Autodesk Inventor part; units mm, degrees
ref_plane "YZ Plane" through (0, 0, 0) normal (1, 0, 0) x (0, 1, 0)
ref_plane "XZ Plane" through (0, 0, 0) normal (0, 1, 0) x (-1, 0, 0)
ref_plane "XY Plane" through (0, 0, 0) normal (0, 0, 1) x (1, 0, 0)
sketch "スケッチ1" plane through (0, 0, 0) normal (0, 1, 0) x (-1, 0, 0)
  line L0 (-8, 10) -> (8, 10)
  line L1 (8, 10) -> (8, -10)
  line L2 (8, -10) -> (-8, -10)
  line L3 (-8, -10) -> (-8, 10)
  line L4 (-8, 10) -> (8, -10) construction
  line L5 (8, 10) -> (-8, -10) construction
  circle A0 centre (0, 15) radius 5
  circle A1 centre (0, -15) radius 5
  line L6 (4.4944, 17.191) -> (8, 10)
  line L7 (-8, 10) -> (-4.4944, 17.191)
  line L8 (4.4944, -17.191) -> (8, -10)
  line L9 (-8, -10) -> (-4.4944, -17.191)
  point P0 (0, 0)
  dimension "d0" = 16
  dimension "d1" = 20
  dimension "d2" = 10
  dimension "d3" = 10
extrude "押し出し1" add sketch "スケッチ1" along normal blind 6.5
sketch "スケッチ2" plane through (0, 6.5, 0) normal (0, 1, 0) x (1, 0, 0)
  line L0 (5.25, -7.8) -> (-5.25, -7.8)
  line L1 (-5.25, -7.8) -> (-5.25, 7.8)
  line L2 (-5.25, 7.8) -> (5.25, 7.8)
  line L3 (5.25, 7.8) -> (5.25, -7.8)
  line L4 (5.25, -7.8) -> (-5.25, 7.8) construction
  line L5 (-5.25, -7.8) -> (5.25, 7.8) construction
  point P0 (0, 0)
  dimension "d6" = 10.5
  dimension "d7" = 15.6
extrude "押し出し2" cut sketch "スケッチ2" against normal blind 1.8
sketch "スケッチ3" plane through (0, 4.7, 0) normal (0, 1, 0) x (1, 0, 0)
  line L0 (-5.25, 7.8) -> (5.25, 7.8)
  line L1 (-5.25, -7.8) -> (-5.25, 7.8)
  line L2 (5.25, -7.8) -> (-5.25, -7.8)
  line L3 (5.25, 7.8) -> (5.25, -7.8)
  line L4 (-5.25, -7.8) -> (-3.65, -7.8)
  line L5 (-3.65, -7.8) -> (-3.65, -6.2)
  line L6 (-3.65, -6.2) -> (-5.25, -6.2)
  line L7 (-5.25, -6.2) -> (-5.25, -7.8)
  line L8 (5.25, -7.8) -> (3.65, -7.8)
  line L9 (3.65, -7.8) -> (3.65, -6.2)
  line L10 (3.65, -6.2) -> (5.25, -6.2)
  line L11 (5.25, -6.2) -> (5.25, -7.8)
  line L12 (-5.25, 7.8) -> (-3.65, 7.8)
  line L13 (-3.65, 7.8) -> (-3.65, 6.2)
  line L14 (-3.65, 6.2) -> (-5.25, 6.2)
  line L15 (-5.25, 6.2) -> (-5.25, 7.8)
  line L16 (-5.25, 7.8) -> (5.25, 7.8)
  line L17 (5.25, 7.8) -> (3.65, 7.8)
  line L18 (3.65, 7.8) -> (3.65, 6.2)
  line L19 (3.65, 6.2) -> (5.25, 6.2)
  line L20 (5.25, 6.2) -> (5.25, 7.8)
  point P0 (0, 0)
  point P1 (-5.25, 6.2)
  point P2 (3.65, -7.8)
  dimension "d10" = 1.6
  dimension "d11" = 1.6
  dimension "d12" = 1.6
  dimension "d13" = 1.6
  dimension "d14" = 1.6
  dimension "d15" = 1.6
  dimension "d16" = 1.6
  dimension "d17" = 1.6
extrude "押し出し3" cut sketch "スケッチ3" against normal blind 3.9 contours L0 L18 L19 L3 L10 L9 L2 L5 L6 L1 L14 L13
sketch "スケッチ4" plane through (0, 6.5, 0) normal (0, 1, 0) x (1, 0, 0)
  arc A0 (-4.4944, -17.191) -> (4.4944, -17.191) centre (0, -15) ccw
  arc A1 (4.4944, 17.191) -> (-4.4944, 17.191) centre (0, 15) ccw
  point P0 (0, 0)
hole "穴1" at (0, 6.5, 15) at (0, 6.5, -15) direction (0, -1, 0) diameter 3.5 end through all
fillet "フィレット1" radius 2 4 edges at (8, 3.25, 10) (8, 3.25, -10) (-8, 3.25, -10) (-8, 3.25, 10)
sketch "スケッチ5" plane through (0, 0, 0) normal (0, -1, 0) x (1, 0, 0)
  line L0 (3.9393, 10.9499) -> (3.9393, -11.5207) construction
  line L1 (3.9393, -11.5207) -> (-3.7897, -11.5207) construction
  line L2 (-3.7897, -11.5207) -> (-3.7897, 10.9499) construction
  line L3 (-3.7897, 10.9499) -> (3.9393, 10.9499) construction
  line L4 (-3.0607, 6.887) -> (-3.0607, 10.9842)
  line L5 (-3.0607, 10.9842) -> (-1.8207, 10.6984)
  line L6 (-1.8207, 10.6984) -> (-1.8207, 9.5556)
  line L7 (-1.8207, 9.5556) -> (2.6993, 8.5156)
  line L8 (2.6993, 8.5156) -> (2.6993, 9.6584)
  line L9 (2.6993, 9.6584) -> (3.9393, 9.367)
  line L10 (3.9393, 9.367) -> (3.9393, 5.2699)
  line L11 (3.9393, 5.2699) -> (2.6993, 5.5556)
  line L12 (2.6993, 5.5556) -> (2.6993, 6.6984)
  line L13 (2.6993, 6.6984) -> (-1.8207, 7.7442)
  line L14 (-1.8207, 7.7442) -> (-1.8207, 6.6013)
  line L15 (-1.8207, 6.6013) -> (-3.0607, 6.887)
  line L16 (-3.0607, -1.9358) -> (-3.0607, -0.1301)
  line L17 (-3.0607, -0.1301) -> (1.5164, -1.1873)
  line L18 (1.5164, -1.1873) -> (-1.415, 0.7327)
  line L19 (-1.415, 0.7327) -> (-1.415, 1.9784)
  line L20 (-1.415, 1.9784) -> (1.7107, 2.6013)
  line L21 (1.7107, 2.6013) -> (-3.0607, 3.6984)
  line L22 (-3.0607, 3.6984) -> (-3.0607, 5.4127)
  line L23 (-3.0607, 5.4127) -> (3.9393, 3.7956)
  line L24 (3.9393, 3.7956) -> (3.9393, 1.7213)
  line L25 (3.9393, 1.7213) -> (0.425, 0.9556)
  line L26 (0.425, 0.9556) -> (3.9393, -1.4216)
  line L27 (3.9393, -1.4216) -> (3.9393, -3.553)
  line L28 (3.9393, -3.553) -> (-3.0607, -1.9358)
  line L29 (3.9393, -11.473) -> (-0.4322, -10.4558)
  spline S0 degree 2 poles (-0.4322, -10.4558) (-1.8836, -10.113) (-3.1979, -8.4787) (-3.1979, -6.9244) knots 0 0 0 1 2 2 2
  spline S1 degree 2 poles (-3.1979, -6.9244) (-3.1979, -5.5416) (-2.2036, -4.1244) (-1.1979, -4.1244) knots 0 0 0 1 2 2 2
  spline S2 degree 2 poles (-1.1979, -4.1244) (-0.9922, -4.1244) (-0.5693, -4.193) (-0.3979, -4.2273) knots 0 0 0 1 2 2 2
  line L30 (-0.3979, -4.2273) -> (3.9393, -5.2387)
  line L31 (3.9393, -5.2387) -> (3.9393, -7.0616)
  line L32 (3.9393, -7.0616) -> (-0.4036, -6.0501)
  spline S3 degree 2 poles (-0.4036, -6.0501) (-0.535, -6.0158) (-0.8493, -5.9758) (-0.9522, -5.9758) knots 0 0 0 1 2 2 2
  spline S4 degree 2 poles (-0.9522, -5.9758) (-1.3922, -5.9758) (-1.8493, -6.5073) (-1.8493, -7.1244) knots 0 0 0 1 2 2 2
  spline S5 degree 2 poles (-1.8493, -7.1244) (-1.8493, -7.7187) (-1.1922, -8.4558) (-0.495, -8.6158) knots 0 0 0 1 2 2 2
  line L33 (-0.495, -8.6158) -> (3.9393, -9.6501)
  line L34 (3.9393, -9.6501) -> (3.9393, -11.473)
  point P0 (0, 0)
extrude "押し出し4" cut sketch "スケッチ5" against normal blind 0.4
equation "\"d3\" = d2"
properties part number "3D_bno055_top_3D プリント"
Source: CAD feature listing. Evaluate the final solid. Frame: model axes, mm. A direction names the side the tool comes from. Give positions to 0.01 mm unless a question says otherwise; leave off trailing zeros. Write each loop counter-clockwise with the first axis right and the second up, starting at its lowest first coordinate (ties: lowest second). Pieces come first, ordered by that corner, then holes. Notation, with made-up numbers: M 89,82 L 134,82 A35 ccw 134,116 Z; hole C -20.75,53 d9. An arc over 180 degrees is marked long. Return JSON: item names as keys, results as strings. Group by question number.
1) Pull-direction query (X, two-part tool) for faces 4 (the face through (6.169, 3.204, 13.755)), 5 (the face through (1.74, 0.197, -4.726)), 6 (the face through (0, 3, 20)); classes: pulls with the +X half, pulls with the -X half, needs draft (parallel to the pull), parting line crosses it, or undercut.
2) Pin query (flat end, axial travel): P1, Ø3, axis at y = 3, z = 13, coming from the -X side; P2, Ø0.8, axis at x = 4.5, y = 2, coming from the -Z side; P3, Ø0.5, axis at x = 4.5, z = -6.5, coming from the +Y side. Return the tip coordinate at first contact, or that it passes through.
3) Cut plane B-B, the plane z = -15. Output: boundary loops of the cut face in (x, y).
4) Material intervals for line 1 along Z through (x, y) = (0, 4.75); line 2 along Z through (x, y) = (1.25, 0.5); line 3 along Y through (x, z) = (-2, 9), sorted ascending. Write a range as [from, to].
5) Cut plane C-C, the plane x = 0. Give the number of separate pieces and of enclosed holes in the cut face, plus the area to 3 significant figures.
6) Cut plane D-D, the plane z = 12.5. Output: boundary loops of the cut face in (x, y).
7) Cut plane A-A, the plane y = 5.5. Output: boundary loops of the cut face in (x, z).
8) Set-up query: faces 1 (the face through (7.95, 3.3, 9.99)), 2 (the face through (0.471, 0.197, 7.214)), 3 (the face through (-3.65, 3, 7)). Return all of +Z, -Z, +X, -X, +Y, -Y with unobstructed straight access to the full face (end or side cutting, diameter ignored); none if empty.
Recorded:
{
 "1": {"face 4": "pulls with the +X half", "face 5": "undercut", "face 6": "parting line crosses it"},
 "2": {"P1": "stops at x = -7.27", "P2": "stops at z = -17.86", "P3": "stops at y = 4.7"},
 "3": {"outline": "M -5.56,0 L -1.75,0 L -1.75,6.5 L -5.56,6.5 Z; M 1.75,0 L 5.56,0 L 5.56,6.5 L 1.75,6.5 Z"},
 "4": {"line 1": "z = [-20, -16.75], [-13.25, -7.8], [7.8, 13.25], [16.75, 20]", "line 2": "z = [-19.84, -16.22], [-13.78, 13.78], [16.22, 19.84]", "line 3": "y = [0.4, 6.5]"},
 "5": {"separate pieces": "3", "enclosed holes": "0", "area": "121 mm²"},
 "6": {"outline": "M -6.78,0 L 6.78,0 L 6.78,6.5 L -6.78,6.5 Z"},
 "7": {"outline": "M -8,-9.54 A2 ccw -7.8,-10.41 L -4.49,-17.19 A5 ccw 4.49,-17.19 L 7.8,-10.41 A2 ccw 8,-9.54 L 8,9.54 A2 ccw 7.8,10.41 L 4.49,17.19 A5 ccw -4.49,17.19 L -7.8,10.41 A2 ccw -8,9.54 Z; hole M -5.25,-7.8 L 5.25,-7.8 L 5.25,7.8 L -5.25,7.8 Z; hole C 0,-15 d3.5; hole C 0,15 d3.5"},
 "8": {"face 1": "+Z, +X, +Y, -Y", "face 2": "-Y", "face 3": "+Y"}
}
